Autodesk Inventor part; units mm, degrees
ref_plane "YZ Plane" through (0, 0, 0) normal (1, 0, 0) x (0, 1, 0)
ref_plane "XZ Plane" through (0, 0, 0) normal (0, 1, 0) x (-1, 0, 0)
ref_plane "XY Plane" through (0, 0, 0) normal (0, 0, 1) x (1, 0, 0)
sketch "Sketch1" plane through (0, 0, 0) normal (0, 0, 1) x (1, 0, 0)
  line L0 (-36, 52.5) -> (36, 52.5)
  line L1 (36, 52.5) -> (36, -52.5)
  line L2 (36, -52.5) -> (-36, -52.5)
  line L3 (-36, -52.5) -> (-36, 52.5)
  line L4 (-36, 52.5) -> (36, -52.5) construction
  line L5 (36, 52.5) -> (-36, -52.5) construction
  circle A0 centre (31.1, -37.5) radius 1.6
  line L6 (0, 0) -> (12.8976, 0)
  line L7 (0, 0) -> (0, 11.3109)
  circle A1 centre (-31.1, -37.5) radius 1.6
  circle A2 centre (31.1, 37.5) radius 1.6
  circle A3 centre (-31.1, 37.5) radius 1.6
  circle A4 centre (-31, -46.5) radius 1.6
  circle A5 centre (-31, 46.5) radius 1.6
  circle A6 centre (31, -46.5) radius 1.6
  circle A7 centre (31, 46.5) radius 1.6
  dimension "d0" = 72
  dimension "d1" = 105
  dimension "d2" = 3.2
  dimension "d3" = 4.9
  dimension "d4" = 15
  dimension "d6" = 3.2
  dimension "d7" = 6
  dimension "d8" = 5
extrude "Plate1" add sketch "Sketch1" along normal blind 1
sketch "Sketch2" plane through (0, 0, 1) normal (0, 0, 1) x (1, 0, 0)
  line L0 (-17.5, 30) -> (-12.5, 30)
  line L1 (-7.5, 25) -> (-7.5, 10)
  line L2 (-12.5, 5) -> (-17.5, 5)
  line L3 (-22.5, 10) -> (-22.5, 25)
  line L4 (-22.5, 30) -> (-7.5, 5) construction
  line L5 (-7.5, 30) -> (-22.5, 5) construction
  line L6 (-28.3073, 0) -> (28.3073, 0)
  line L7 (0, 37.5) -> (0, -37.5)
  arc A0 (-17.5, 30) -> (-22.5, 25) centre (-17.5, 25) ccw
  arc A1 (-7.5, 25) -> (-12.5, 30) centre (-12.5, 25) ccw
  arc A2 (-12.5, 5) -> (-7.5, 10) centre (-12.5, 10) ccw
  arc A3 (-22.5, 10) -> (-17.5, 5) centre (-17.5, 10) ccw
  line L8 (17.5, 30) -> (12.5, 30)
  line L9 (7.5, 25) -> (7.5, 10)
  line L10 (12.5, 5) -> (17.5, 5)
  line L11 (22.5, 10) -> (22.5, 25)
  line L12 (22.5, 30) -> (7.5, 5) construction
  line L13 (7.5, 30) -> (22.5, 5) construction
  arc A4 (22.5, 25) -> (17.5, 30) centre (17.5, 25) ccw
  arc A5 (12.5, 30) -> (7.5, 25) centre (12.5, 25) ccw
  arc A6 (7.5, 10) -> (12.5, 5) centre (12.5, 10) ccw
  arc A7 (17.5, 5) -> (22.5, 10) centre (17.5, 10) ccw
  line L14 (-17.5, -30) -> (-12.5, -30)
  line L15 (-7.5, -25) -> (-7.5, -10)
  line L16 (-12.5, -5) -> (-17.5, -5)
  line L17 (-22.5, -10) -> (-22.5, -25)
  line L18 (-22.5, -30) -> (-7.5, -5) construction
  line L19 (-7.5, -30) -> (-22.5, -5) construction
  arc A8 (-22.5, -25) -> (-17.5, -30) centre (-17.5, -25) ccw
  arc A9 (-12.5, -30) -> (-7.5, -25) centre (-12.5, -25) ccw
  arc A10 (-7.5, -10) -> (-12.5, -5) centre (-12.5, -10) ccw
  arc A11 (-17.5, -5) -> (-22.5, -10) centre (-17.5, -10) ccw
  arc A12 (7.5, -25) -> (12.5, -30) centre (12.5, -25) ccw
  line L20 (7.5, -25) -> (7.5, -10)
  line L21 (17.5, -30) -> (12.5, -30)
  arc A13 (17.5, -30) -> (22.5, -25) centre (17.5, -25) ccw
  arc A14 (12.5, -5) -> (7.5, -10) centre (12.5, -10) ccw
  line L22 (22.5, -10) -> (22.5, -25)
  arc A15 (22.5, -10) -> (17.5, -5) centre (17.5, -10) ccw
  line L23 (7.5, -30) -> (22.5, -5) construction
  line L24 (22.5, -30) -> (7.5, -5) construction
  line L25 (12.5, -5) -> (17.5, -5)
  point P0 (0, 0)
  point P1 (-15, 17.5)
  point P2 (0, 0)
  point P3 (15, 17.5)
  point P4 (-15, -17.5)
  point P5 (15, -17.5)
  dimension "d9" = 15
  dimension "d10" = 25
  dimension "d12" = 10
  dimension "d13" = 15
  dimension "d14" = 5
extrude "Cut1" cut sketch "Sketch2" against normal blind 1
equation "\"d15\" = 厚度"
equation "\"d5\" = 厚度"
equation "\"折彎半徑\" = 厚度"
equation "\"折彎離隙寬度\" = 厚度"
equation "\"折彎離隙深度\" = 0.5 * 厚度"
equation "\"轉角離隙大小\" = 4 * 厚度"
equation "\"最小剩餘\" = 2 * 厚度"
equation "\"轉移半徑\" = 折彎半徑"
equation "\"Jacobi半徑大小\" = 折彎半徑"
equation "\"間隙大小\" = 厚度"
properties part number "battery_box_24V_side1" material "Aluminum"
For this review, take the finished solid that the model builds, in its own axes (mm). Round coordinates to 2 decimals unless told otherwise and drop trailing zeros. Order: outer loops, then holes, each group sorted by start corner. A loop starts at its lowest first (then second) coordinate and runs counter-clockwise, first axis right, second up. Notation, with made-up numbers: M -25,-3.5 L 20,-3.5 A34 ccw 20,30.5 Z; hole C 77.25,-31.5 d4. An arc over 180 degrees is marked long. Use a Markdown table: item, result. Add a question column.
Item 1: Add section A-A, the plane y = -15. Give the boundary of the cut face in (x, z).
Item 2: To check wall thickness, follow line 1 along Y through (x, z) = (31, 0.3); line 2 along X through (y, z) = (-21, 0.7); line 3 along Y through (x, z) = (-14, 0.4). State the ranges of each line that lie inside material, in increasing order.
Item 3: Add section C-C, the plane x = -31.1. Give the boundary of the cut face in (y, z), then the cut area to 3 significant figures.
Item 4: Add section B-B, the plane x = -15.5. Give the boundary of the cut face in (y, z).
Item 5: Insertion check: pin 1 (3.5 mm diameter, centred on x = -31.1, y = 37.5, fed in from +Z). The pin has a flat end and moves straight along its axis. Give the tip position at first contact, or say it passes through.
Item 6: Mouldability with a two-part tool opening along Y and no side actions: class faces 1 (the flat face through (-1, 1, 1)), 2 (the cylindrical face through (8.93, -28.5, 0.51)) as released by +Y, released by -Y, zero draft, split by the parting line, or undercut.
Item 7: Add section D-D, the plane z = 0.35. State how many separate pieces and enclosed holes the cut face has, then the cut area to 3 significant figures.
Geometry results:
| question | item | result |
|---|---|---|
| 1 | outline | M -36,0 L -22.5,0 L -22.5,1 L -36,1 Z; M -7.5,0 L 7.5,0 L 7.5,1 L -7.5,1 Z; M 22.5,0 L 36,0 L 36,1 L 22.5,1 Z |
| 2 | line 1 | y = -52.5 to -48.1, -44.9 to -39.1, -35.9 to 35.9, 39.1 to 44.9, 48.1 to 52.5 |
| 2 | line 2 | x = -36 to -22.5, -7.5 to 7.5, 22.5 to 36 |
| 2 | line 3 | y = -52.5 to -30, -5 to 5, 30 to 52.5 |
| 3 | outline | M -52.5,0 L -48.1,0 L -48.1,1 L -52.5,1 Z; M -44.9,0 L -39.1,0 L -39.1,1 L -44.9,1 Z; M -35.9,0 L 35.9,0 L 35.9,1 L -35.9,1 Z; M 39.1,0 L 44.9,0 L 44.9,1 L 39.1,1 Z; M 48.1,0 L 52.5,0 L 52.5,1 L 48.1,1 Z |
| 3 | area | 92.2 mm² |
| 4 | outline | M -52.5,0 L -30,0 L -30,1 L -52.5,1 Z; M -5,0 L 5,0 L 5,1 L -5,1 Z; M 30,0 L 52.5,0 L 52.5,1 L 30,1 Z |
| 5 | pin 1 | stops at z = 1 |
| 6 | face 1 | zero draft |
| 6 | face 2 | undercut |
| 7 | separate pieces | 1 |
| 7 | enclosed holes | 12 |
| 7 | area | 6,080 mm² |
